Here's how the part is built. I have some questions about the finished solid (model axes, mm). Face numbers are marked on the shaded views. A direction names the side the tool comes from. Give positions to 0.01 mm unless a question says otherwise; leave off trailing zeros. Write each loop counter-clockwise with the first axis right and the second up, starting at its lowest first coordinate (ties: lowest second). Pieces come first, ordered by that corner, then holes. Notation, with made-up numbers: (-21.5, -36) -> (10.5, -36) arc R10 ccw to (10.5, -27) -> close; hole circle Ø9 at (32.5, -31). An arc over 180 degrees is marked (long way). Put each result on its own line as item: value. Start each with the question number.
from build123d import *


with BuildPart() as f3:
    # F3: sweep along a path in F0
    with BuildLine(Plane.XY) as f3_path:
        Line((6.1897202132, 8.5194189943), (26.220075585, 8.5194189943))
        Line((26.220075585, 8.5194189943), (10.0151776859, -3.2541284914))
        Line((10.0151776859, -3.2541284914), (16.2048978991, -22.3041284914))
        Line((16.2048978991, -22.3041284914), (0, -10.5305810057))
        Line((0, -10.5305810057), (-16.2048978991, -22.3041284914))
        Line((-16.2048978991, -22.3041284914), (-10.0151776859, -3.2541284914))
        Line((-10.0151776859, -3.2541284914), (-26.220075585, 8.5194189943))
        Line((-26.220075585, 8.5194189943), (-6.1897202132, 8.5194189943))
        Line((-6.1897202132, 8.5194189943), (0, 27.5694189943))
        Line((0, 27.5694189943), (6.1897202132, 8.5194189943))
    # F2 (on plane+point) → F3 (sweep)
    with BuildSketch(Plane.YZ.offset(6.1897202132)):
        Polygon((7.0194189943, 3.2167603808), (8.5194189943, 0), (10.0194189943, 3.2167603808), (10.0194189943, 12.7), (11.0194189943, 12.7), (11.0194189943, 14.2), (8.5194189943, 14.2), (6.0194189943, 14.2), (6.0194189943, 12.7), (7.0194189943, 12.7), align=None)
    sweep(path=f3_path.line, transition=Transition.RIGHT)


solid = f3.part
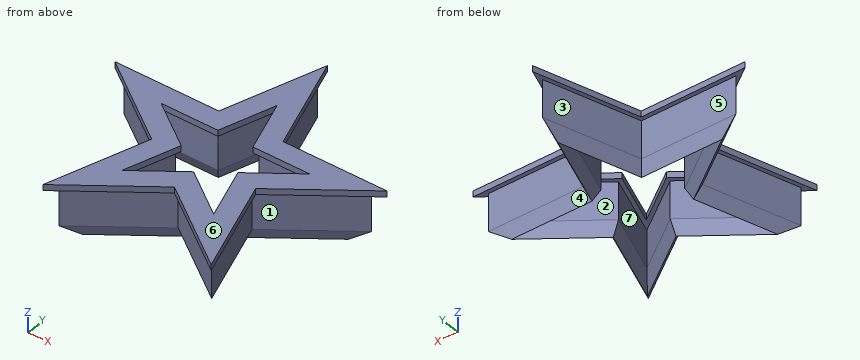
1) Thinking about a two-plate mould opening in Y: for the marked faces 5, 6 and 7, which applies, released by +Y, released by -Y, zero draft, split by the parting line, or undercut?
2) I need wall thicknesses on probe 1 along X at (y, z) = (-13.5, 10.75); probe 2 along Y at (x, z) = (-19.5, 11.5); probe 3 along X at (y, z) = (2, 8). Which ranges of each line are inside material? Lowest first, please.
3) Which directions (+Z, -Z, +X, -X, +Y, -Y) give clear straight access to the entire face, cutting with the end or side of a thin tool? Please do the marked faces 1, 2, 3 and 4.
4) I want a section at B-B, the plane x = 17. Write out the boundary of the cut face in (y, z).
5) I want a section at D-D, the plane x = -1. Write out the boundary of the cut face in (y, z), and give its area (3 significant figures).
6) I want a section at C-C, the plane y = -19.5. Write out the boundary of the cut face in (x, z), and give its area (3 significant figures).
7) I want a section at A-A, the plane z = 7.25. Write out the boundary of the cut face in (x, y), and give its area (3 significant figures).
8) I'm going to push flat-ended pins straight in: pin 1 Ø1 at (y, z) = (16, 10.5) entering from -X; pin 2 Ø1.6 at (x, z) = (-21, 13.5) entering from +Y; pin 3 Ø3 at (x, z) = (-17.5, 2.5) entering from -Y. Where does each tip first touch, or does it pass through?
Established:
1. face 5: released by +Y
1. face 6: zero draft
1. face 7: undercut
2. probe 1: x = -14.92 to -11.77, -6.64 to -1.54, 1.54 to 6.64, 11.77 to 14.92
2. probe 2: y = 1.78 to 5.49, 7.02 to 10.02
2. probe 3: x = -19.8 to -14.69, 14.69 to 19.8
3. face 1: -Z, +X
3. face 2: -Z
3. face 3: -Z, -X, +Y
3. face 4: -Z, +X, +Y
4. outline: (-25.97, 12.7) -> (-24.74, 12.7) -> (-24.74, 3.22) -> (-23.4, 0.9) -> (-19.9, 3.22) -> (-19.9, 12.7) -> (-16.66, 12.7) -> (-16.66, 14.2) -> (-25.97, 14.2) -> close; (-1.27, 12.7) -> (-0.03, 12.7) -> (-0.03, 3.22) -> (1.82, 0) -> (3.67, 3.22) -> (3.67, 12.7) -> (4.91, 12.7) -> (4.91, 14.2) -> (-1.27, 14.2) -> close; (6.02, 12.7) -> (7.02, 12.7) -> (7.02, 3.22) -> (8.52, 0) -> (10.02, 3.22) -> (10.02, 12.7) -> (11.02, 12.7) -> (11.02, 14.2) -> (6.02, 14.2) -> close
5. outline: (-14.35, 12.7) -> (-13.11, 12.7) -> (-13.11, 3.22) -> (-11.26, 0) -> (-9.4, 3.22) -> (-9.4, 12.7) -> (-8.17, 12.7) -> (-8.17, 14.2) -> (-14.35, 14.2) -> close; (16.4, 12.7) -> (19.64, 12.7) -> (19.64, 3.22) -> (24.49, 0) -> (29.35, 3.22) -> (29.35, 12.7) -> (32.58, 12.7) -> (32.58, 14.2) -> (16.4, 14.2) -> close
5. area: 182 mm2
6. outline: (-17.92, 12.7) -> (-16.87, 12.7) -> (-16.87, 3.22) -> (-15.29, 0) -> (-14.17, 2.3) -> (-12.35, 0) -> (-9.79, 3.22) -> (-9.79, 12.7) -> (-8.09, 12.7) -> (-8.09, 14.2) -> (-17.92, 14.2) -> close; (8.09, 12.7) -> (9.79, 12.7) -> (9.79, 3.22) -> (12.35, 0) -> (14.17, 2.3) -> (15.29, 0) -> (16.87, 3.22) -> (16.87, 12.7) -> (17.92, 12.7) -> (17.92, 14.2) -> (8.09, 14.2) -> close
6. area: 189 mm2
7. outline: (-30.84, 10.02) -> (-11.78, -3.83) -> (-19.06, -26.23) -> (0, -12.38) -> (19.06, -26.23) -> (11.78, -3.83) -> (30.84, 10.02) -> (7.28, 10.02) -> (0, 32.42) -> (-7.28, 10.02) -> close; hole (-21.6, 7.02) -> (-8.25, -2.68) -> (-13.35, -18.38) -> (0, -8.68) -> (13.35, -18.38) -> (8.25, -2.68) -> (21.6, 7.02) -> (5.1, 7.02) -> (0, 22.72) -> (-5.1, 7.02) -> close
7. area: 601 mm2
8. pin 1: stops at x = -5.5
8. pin 2: stops at y = 11.02
8. pin 3: stops at y = -26.06
